from build123d import *

# Parameters (mm, degrees)
HOLE_WIZARD_M12_1_D = 10.2


# Read off the part's stored shape, not the designer's step: M16 机械螺纹 螺柱1
with BuildPart() as part:
    # 草图1 → 旋转1 (revolve)
    with BuildSketch(Plane.XY, mode=Mode.PRIVATE) as revolve_1_sk:
        Polygon((5, 0), (5, 35), (8, 35), (8, 33), (11, 33), (11, 30), (7, 30), (7, 29), (8, 29), (8, 0), align=None)
    revolve(revolve_1_sk.sketch.rotate(Axis((0, 0, 0), (0, 1, 0)), 90), axis=Axis((0, 0, 0), (0, 1, 0)))

    # M16 机械螺纹 螺柱1 outline → M16 机械螺纹 螺柱1 (revolve, cut)
    with BuildSketch(Plane.XY):
        Polygon((8, 1.0825), (6.9175, 0), (8, 0), align=None)
    revolve(axis=Axis((0, 0, 0), (0, 1, 0)), mode=Mode.SUBTRACT)

    # M12 螺纹孔1 (through all)
    with Locations(Plane(origin=(0, 35, 0), x_dir=(1, 0, 0), z_dir=(0, 1, 0))):
        with Locations((0, 0)):
            Hole(HOLE_WIZARD_M12_1_D / 2)


solid = part.part
Input: part model. Units: mm. Frame: model coordinates. A direction names the side the tool comes from. Coordinates: 2 decimals unless noted, no trailing zeros. Loops run counter-clockwise (first coordinate to the right, second up) from the corner with the lowest first, then second, coordinate; pieces in that order, holes last. Notation, with made-up numbers: (-13, 51) -> (-5, 51) arc R11 cw to (-5, 62) -> close; hole circle Ø8 at (-4, -20). An arc over 180 degrees is marked (long way). One line per item, written item: value.
(1) Cut plane D-D (z = 9). Output: boundary loops of the cut face in (x, y).
Answer below:
outline: (-6.32, 30) -> (6.32, 30) -> (6.32, 33) -> (-6.32, 33) -> close
(2) Ray query, line 1 along Z through (x, y) = (0, 25); line 2 along Y through (x, z) = (8.5, 4.25); line 3 along Z through (x, y) = (-2.25, 20.5). Return the intervals inside material, ascending.
Answer below:
line 1: z = -8 to -5.1, 5.1 to 8
line 2: y = 30 to 33
line 3: z = -7.68 to -4.58, 4.58 to 7.68
(3) Pin query (flat end, axial travel): pin 1 Ø8 at (y, z) = (8, 2) entering from +X; pin 2 Ø5 at (y, z) = (23.5, -0.5) entering from -X; pin 3 Ø5 at (x, y) = (5, 21.5) entering from +Z. Return the tip coordinate at first contact, or that it passes through.
Answer below:
pin 1: stops at x = 8
pin 2: stops at x = -8
pin 3: stops at z = 7.6
(4) Cut plane B-B (x = 0). Output: boundary loops of the cut face in (y, z), then the cut area to 3 significant figures.
Answer below:
outline: (0, -6.92) -> (1.08, -8) -> (29, -8) -> (29, -7) -> (30, -7) -> (30, -11) -> (33, -11) -> (33, -8) -> (35, -8) -> (35, -5.1) -> (0, -5.1) -> close; (0, 5.1) -> (35, 5.1) -> (35, 8) -> (33, 8) -> (33, 11) -> (30, 11) -> (30, 7) -> (29, 7) -> (29, 8) -> (1.08, 8) -> (0, 6.92) -> close
area: 218 mm2
(5) Cut plane A-A (z = 0). Output: boundary loops of the cut face in (x, y).
Answer below:
outline: (-11, 30) -> (-7, 30) -> (-7, 29) -> (-8, 29) -> (-8, 1.08) -> (-6.92, 0) -> (-5.1, 0) -> (-5.1, 35) -> (-8, 35) -> (-8, 33) -> (-11, 33) -> close; (5.1, 0) -> (6.92, 0) -> (8, 1.08) -> (8, 29) -> (7, 29) -> (7, 30) -> (11, 30) -> (11, 33) -> (8, 33) -> (8, 35) -> (5.1, 35) -> close
(6) Set-up query: faces 4 (the face through (8, 33, -2)), 5 (the face through (-0.2, 30, -7.2)), 6 (the face through (-2.4, 17.3, 4.5)). Return all of +Z, -Z, +X, -X, +Y, -Y with unobstructed straight access to the full face (end or side cutting, diameter ignored); none if empty.
Answer below:
face 4: +Y
face 5: none
face 6: +Y, -Y
(7) Draft query along Y for faces 1 (the face through (7.1, 14.85, -3.69)), 2 (the face through (6, 29, 4)), 3 (the face through (5, 0, 3)). Return one class per face: pulls with the +Y half, pulls with the -Y half, needs draft (parallel to the pull), parting line crosses it, or undercut.
Answer below:
face 1: needs draft
face 2: undercut
face 3: pulls with the -Y half
(8) Cut plane C-C (y = 10). Output: boundary loops of the cut face in (x, z).
Answer below:
outline: circle Ø16 at (0, 0); hole circle Ø10.2 at (0, 0)
